from build123d import *

# Parameters (mm, degrees)
SKETCH1_W           = 100
SKETCH1_H           = 120
BOSS_EXTRUDE1_DEPTH = 2.2
SKETCH2_R           = 10
CUT_EXTRUDE1_DEPTH  = 10
SKETCH3_W           = 100
SKETCH3_H           = 4.205559055
BOSS_EXTRUDE2_DEPTH = 2


with BuildPart() as part:
    # Sketch1 → Boss-Extrude1 (new body)
    with BuildSketch(Plane.XY):
        with Locations((50, 60)):
            Rectangle(SKETCH1_W, SKETCH1_H)
    extrude(amount=BOSS_EXTRUDE1_DEPTH)

    # Sketch2 → Cut-Extrude1 (cut)
    with BuildSketch(Plane.XY.offset(2.2)):
        with Locations((88, 12)):
            Circle(SKETCH2_R)
        with Locations((63, 12)):
            Circle(SKETCH2_R)
        with Locations((38, 12)):
            Circle(SKETCH2_R)
        with Locations((13, 12)):
            Circle(SKETCH2_R)
        with Locations((63, 37)):
            Circle(SKETCH2_R)
        with Locations((38, 37)):
            Circle(SKETCH2_R)
        with Locations((13, 37)):
            Circle(SKETCH2_R)
        with Locations((63, 62)):
            Circle(SKETCH2_R)
        with Locations((38, 62)):
            Circle(SKETCH2_R)
        with Locations((13, 62)):
            Circle(SKETCH2_R)
        with Locations((63, 87)):
            Circle(SKETCH2_R)
        with Locations((38, 87)):
            Circle(SKETCH2_R)
        with Locations((13, 87)):
            Circle(SKETCH2_R)
        with Locations((88, 37)):
            Circle(SKETCH2_R)
        with Locations((88, 62)):
            Circle(SKETCH2_R)
        with Locations((88, 87)):
            Circle(SKETCH2_R)
    extrude(amount=-CUT_EXTRUDE1_DEPTH, mode=Mode.SUBTRACT)

    # Sketch3 → Boss-Extrude2 (add)
    with BuildSketch(Plane.XY.offset(2.2)):
        with Locations((50, 117.897220473)):
            Rectangle(SKETCH3_W, SKETCH3_H)
    extrude(amount=BOSS_EXTRUDE2_DEPTH)


solid = part.part
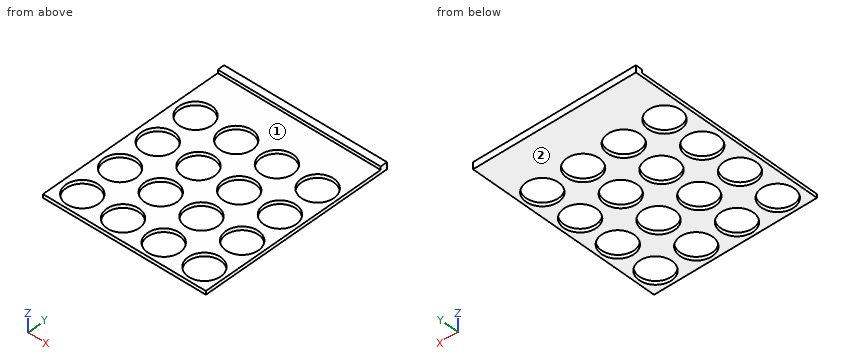
Work out the finished part from the listing and answer in its coordinate system (mm). Face numbers are marked on the shaded views. A direction names the side the tool comes from. Round coordinates to 2 decimals unless told otherwise and drop trailing zeros. Write each loop counter-clockwise with the first axis right and the second up, starting at its lowest first coordinate (ties: lowest second). Pieces come first, ordered by that corner, then holes. Notation, with made-up numbers: M 68,84.5 L 104,84.5 A28 ccw 104,111.5 Z; hole C 30.25,-38.75 d1. An arc over 180 degrees is marked long. Use a Markdown table: item, result.
1) The part is cut by section D-D on y = 112. Give the vertices of the cut face in (x, z), plus the area to 3 significant figures.
Taken from the geometry:
| item | result |
|---|---|
| outline | M 0,0 L 100,0 L 100,2.2 L 0,2.2 Z |
| area | 220 mm2 |
2) Flat-ended cylindrical pins translate along their axes: pin 1 (18 mm diameter, centred on x = 88, y = 12, fed in from -Z); pin 2 (0.6 mm diameter, centred on x = 71, z = 3.5, fed in from -Y); pin 3 (8 mm diameter, centred on x = 12.5, y = 71.5, fed in from +Z). Find the tip coordinate at first contact, or state that the pin passes through.
Taken from the geometry:
| item | result |
|---|---|
| pin 1 | passes through |
| pin 2 | stops at y = 115.79 |
| pin 3 | stops at z = 2.2 |
3) The part is cut by section C-C on x = 85.5. Give the vertices of the cut face in (y, z).
Taken from the geometry:
| item | result |
|---|---|
| outline | M 0,0 L 2.32,0 L 2.32,2.2 L 0,2.2 Z; M 21.68,0 L 27.32,0 L 27.32,2.2 L 21.68,2.2 Z; M 46.68,0 L 52.32,0 L 52.32,2.2 L 46.68,2.2 Z; M 71.68,0 L 77.32,0 L 77.32,2.2 L 71.68,2.2 Z; M 96.68,0 L 120,0 L 120,4.2 L 115.79,4.2 L 115.79,2.2 L 96.68,2.2 Z |
4) The part is cut by section B-B on z = 1.55. State how many separate pieces and enclosed holes the cut face has, plus the area to 3 significant figures.
Taken from the geometry:
| item | result |
|---|---|
| separate pieces | 1 |
| enclosed holes | 16 |
| area | 6,970 mm2 |
5) Consider line 1 (Y direction, x = 63, z = 0.6); line 2 (Y direction, x = 47, z = 1.2); line 3 (X direction, y = 64, z = 1.95). Determine where each line is inside the solid, lowest interval first. Write a range as [from, to].
Taken from the geometry:
| item | result |
|---|---|
| line 1 | y = [0, 2], [22, 27], [47, 52], [72, 77], [97, 120] |
| line 2 | y = [0, 7.64], [16.36, 32.64], [41.36, 57.64], [66.36, 82.64], [91.36, 120] |
| line 3 | x = [0, 3.2], [22.8, 28.2], [47.8, 53.2], [72.8, 78.2], [97.8, 100] |
6) The part is cut by section A-A on y = 87. Give the vertices of the cut face in (x, z).
Taken from the geometry:
| item | result |
|---|---|
| outline | M 0,0 L 3,0 L 3,2.2 L 0,2.2 Z; M 23,0 L 28,0 L 28,2.2 L 23,2.2 Z; M 48,0 L 53,0 L 53,2.2 L 48,2.2 Z; M 73,0 L 78,0 L 78,2.2 L 73,2.2 Z; M 98,0 L 100,0 L 100,2.2 L 98,2.2 Z |
7) Which of the six approach directions +Z, -Z, +X, -X, +Y, -Y give full straight-line access (tool end or side, diameter ignored) to the marked faces 1 and 2?
Taken from the geometry:
| item | result |
|---|---|
| face 1 | +Z, +X, -X, -Y |
| face 2 | -Z, +X, -X, +Y, -Y |
